Geometry: final body of the model. Coordinates: model frame, mm. Face numbers are marked on the shaded views. A direction names the side the tool comes from. Coordinates: 2 decimals unless noted, no trailing zeros. Write each loop counter-clockwise with the first axis right and the second up, starting at its lowest first coordinate (ties: lowest second). Pieces come first, ordered by that corner, then holes.
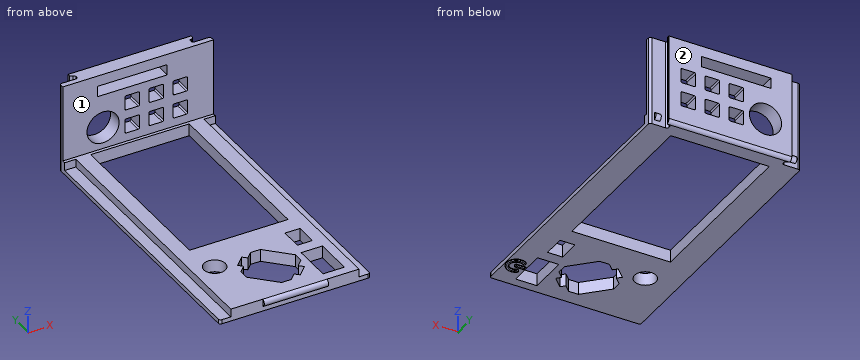
from build123d import *

# Parameters (mm, degrees)
SKETCH_2_W                     = 2.80320188
SKETCH_2_H                     = 4.10319928
SKETCH_2_R                     = 2
SKETCH_2_W_2                   = 3.99999908
SKETCH_2_H_2                   = 7.20319816
EXTRUDE_1_DEPTH                = 2.3
EXTRUDE_2_DEPTH                = 14.4
EXTRUDE_2_DEPTH_BACK           = 2.3
SKETCH_3_W                     = 28.14
SKETCH_3_H                     = 3.4
SKETCH_4_R                     = 3
CUT_EXTRUDE_1_DEPTH            = 3.4
SKETCH_2_3_W                   = 2.1
SKETCH_2_3_H                   = 50.95
CUT_EXTRUDE_2_DEPTH            = 1.5
CUT_EXTRUDE_3_REACH            = 62.506
SKETCH_7_W                     = 28.14
SKETCH_7_H                     = 0.6
SKETCH_8_W                     = 13
SKETCH_8_H                     = 2
CUT_EXTRUDE_4_DEPTH            = 2.8
CUT_EXTRUDE_5_DEPTH            = 16.7
EXTRUDE_3_DEPTH                = 1
EXTRUDE_4_DEPTH                = 6
EXTRUDE_4_DEPTH_BACK           = 6
FILLET_1_R                     = 0.4
FILLET_2_R                     = 0.7
FILLET_3_R                     = 0.4
SKETCH_12_W                    = 2.753
SKETCH_12_H                    = 2.75
CUT_EXTRUDE_6_DEPTH            = 2.8
FILLET_4_R                     = 0.25
PATTERN_LINEAR_1_COUNT         = 3
PATTERN_LINEAR_1_PITCH         = 4.5
PATTERN_LINEAR_1_COUNT_DIR2    = 2
PATTERN_LINEAR_1_PITCH_DIR2    = 4.5
FILLET_4_OF_PATTERN_LINEAR_1_R = 0.25
EXTRUDE_5_DEPTH                = 0.3
FILLET_6_R                     = 0.3
FILLET_5_R                     = 0.15


with BuildPart() as part:
    # 草图2 → 凸台-拉伸1 (new body)
    with BuildSketch(Plane.XY):
        Polygon((-0.1, 0), (-0.1, -50.95), (28.04, -50.95), (28.04, 0), (23.17, 0), (23.17, -32.5), (4.77, -32.5), (4.77, 0), align=None)
        with Locations((22.14500143, -37.80800287)):
            Rectangle(SKETCH_2_W, SKETCH_2_H, mode=Mode.SUBTRACT)
        with Locations((5.9182, -38.735)):
            Circle(SKETCH_2_R, mode=Mode.SUBTRACT)
        Polygon((19.066193866, -43.992617401), (17.88030086, -45.178511502), (18.608616214, -45.906826856), (16.798423264, -47.717019806), (16.070108746, -46.988705288), (14.884217409, -48.174597721), (13.055787589, -48.174595399), (8.873804338, -43.992612148), (8.873804338, -42.164191444), (10.05969962, -40.978296162), (9.331380194, -40.249976736), (11.141573144, -38.439783786), (11.86989257, -39.168103212), (13.055787589, -37.982208193), (14.884217273, -37.982205871), (19.066193866, -42.164182464), align=None, mode=Mode.SUBTRACT)
        with Locations((22.16999884, -45.67000137)):
            Rectangle(SKETCH_2_W_2, SKETCH_2_H_2, mode=Mode.SUBTRACT)
    extrude(amount=-EXTRUDE_1_DEPTH)

    # 草图3 → 凸台-拉伸2 (add, two sides: drawn at the far end of the back side and taken through both)
    with BuildSketch(Plane.XY.offset(-EXTRUDE_2_DEPTH_BACK)):
        with Locations((13.97, 1.7)):
            Rectangle(SKETCH_3_W, SKETCH_3_H)
    extrude(amount=EXTRUDE_2_DEPTH + EXTRUDE_2_DEPTH_BACK)

    # 草图4 → 切除-拉伸1 (cut)
    with BuildSketch(Plane(origin=(0, 3.4, 0), x_dir=(1, 0, 0), z_dir=(0, 1, 0))):
        with Locations(Location((7.41680127, -4.1, 0), (0, 0, 270))):
            Circle(SKETCH_4_R)
    extrude(amount=-CUT_EXTRUDE_1_DEPTH, mode=Mode.SUBTRACT)

    # 草图2<3> → 切除-拉伸2 (cut)
    with BuildSketch(Plane.XY):
        with Locations((0.95, -25.475)):
            Rectangle(SKETCH_2_3_W, SKETCH_2_3_H)
        with Locations((26.99, -25.475)):
            Rectangle(SKETCH_2_3_W, SKETCH_2_3_H)
    extrude(amount=-CUT_EXTRUDE_2_DEPTH, mode=Mode.SUBTRACT)

    # 切除-拉伸3: up to this face of the body (flat: up to its plane)
    cut_extrude_3_end = Plane(part.part.faces().sort_by_distance((13.97, -33.062941036, 0))[0])
    # 草图7 → 切除-拉伸3 (cut, up to the picked face)
    with BuildSketch(Plane.XY.offset(14.4), mode=Mode.PRIVATE) as cut_extrude_3_sk1:
        with Locations((13.97, 0.3)):
            Rectangle(SKETCH_7_W, SKETCH_7_H)
    cut_extrude_3_tool1 = split(extrude(cut_extrude_3_sk1.sketch, amount=-CUT_EXTRUDE_3_REACH, mode=Mode.PRIVATE), bisect_by=cut_extrude_3_end, keep=Keep.BOTH, mode=Mode.PRIVATE)
    add(cut_extrude_3_tool1.solids().sort_by(Axis((13.97, 0.3, 14.4), (0, 0, -1)))[0], mode=Mode.SUBTRACT)

    # 草图8 → 切除-拉伸4 (cut)
    with BuildSketch(Plane.XZ.offset(-0.6)):
        with Locations((12.9, 11.4)):
            Rectangle(SKETCH_8_W, SKETCH_8_H)
    extrude(amount=-CUT_EXTRUDE_4_DEPTH, mode=Mode.SUBTRACT)

    # 草图9 → 切除-拉伸5 (cut)
    with BuildSketch(Plane.XY.offset(14.4)):
        Polygon((2.5, 2.6), (3.3, 2.6), (3.3, 1.6), (-0.1, 1.6), (-0.1, 3.4), (2.5, 3.4), align=None)
        Polygon((28.04, 3.4), (25.44, 3.4), (25.44, 2.6), (24.64, 2.6), (24.64, 1.6), (28.04, 1.6), align=None)
    extrude(amount=-CUT_EXTRUDE_5_DEPTH, mode=Mode.SUBTRACT)

    # 草图10 → 凸台-拉伸3 (add)
    with BuildSketch(Plane.ZY.offset(-0.8)):
        with BuildLine():
            Line((-1.4, 1.6), (0, 1.6))
            ThreePointArc((0, 1.6), (-0.7, 2.1), (-1.4, 1.6))
        make_face()
    extrude_3 = extrude(amount=-EXTRUDE_3_DEPTH)

    # 镜向1: 凸台-拉伸3 across plane
    add(extrude_3.mirror(Plane.ZY.offset(-13.97)))

    # 草图11 → 凸台-拉伸4 (add, two sides: drawn at the far end of the back side and taken through both)
    with BuildSketch(Plane.ZY.offset(-13.97).offset(-EXTRUDE_4_DEPTH_BACK)):
        with BuildLine():
            Line((-1.4, -50.95), (0, -50.95))
            ThreePointArc((0, -50.95), (-0.7, -51.45), (-1.4, -50.95))
        make_face()
    extrude(amount=EXTRUDE_4_DEPTH + EXTRUDE_4_DEPTH_BACK)

    # 圆角1
    fillet_1_edges = [part.edges().sort_by_distance(p)[0] for p in [
        (3.3, 1.6, 6.05),
        (3.3, 2.6, 6.05),
        (2.5, 2.6, 6.05),
        (24.64, 1.6, 6.05),
        (24.64, 2.6, 6.05),
        (25.44, 2.6, 6.05),
    ]]
    fillet(fillet_1_edges, radius=FILLET_1_R - 0.0001)  # a hair under: the kernel refuses the full size

    # 圆角2
    fillet_2_edges = [part.edges().sort_by_distance(p)[0] for p in [
        (13.97, 3.4, -2.3),
    ]]
    fillet(fillet_2_edges, radius=FILLET_2_R)

    # 圆角3
    fillet_3_edges = [part.edges().sort_by_distance(p)[0] for p in [
        (28.04, 1.6, 6.05),
        (-0.1, 1.6, 6.05),
        (-0.1, -50.95, -1.9),
        (28.04, -50.95, -1.9),
    ]]
    fillet(fillet_3_edges, radius=FILLET_3_R)

    # 草图12 → 切除-拉伸6 (cut)
    with BuildSketch(Plane(origin=(0, 3.4, 0), x_dir=(1, 0, 0), z_dir=(0, 1, 0))):
        with Locations((21.8635, -2.975)):
            Rectangle(SKETCH_12_W, SKETCH_12_H)
    cut_extrude_6 = extrude(amount=-CUT_EXTRUDE_6_DEPTH, mode=Mode.SUBTRACT)

    # 圆角4
    fillet_4_edges = [part.edges().sort_by_distance(p)[0] for p in [
        (23.24, 2, 1.6),
        (23.24, 2, 4.35),
        (20.487, 2, 4.35),
        (20.487, 2, 1.6),
    ]]
    fillet(fillet_4_edges, radius=FILLET_4_R)

    # 阵列(线性)1: Cut-Extrude 6 3 × 2
    with Locations(*[(-i * PATTERN_LINEAR_1_PITCH, 0, j * PATTERN_LINEAR_1_PITCH_DIR2) for i in range(PATTERN_LINEAR_1_COUNT) for j in range(PATTERN_LINEAR_1_COUNT_DIR2) if (i, j) != (0, 0)]):
        add(cut_extrude_6, mode=Mode.SUBTRACT)

    # 圆角4 of 阵列(线性)1
    fillet_4_of_pattern_linear_1_edges = [part.edges().sort_by_distance(p)[0] for p in [
        (23.24, 2, 6.1),
        (23.24, 2, 8.85),
        (20.487, 2, 8.85),
        (20.487, 2, 6.1),
        (18.74, 2, 1.6),
        (18.74, 2, 4.35),
        (15.987, 2, 4.35),
        (15.987, 2, 1.6),
        (18.74, 2, 6.1),
        (18.74, 2, 8.85),
        (15.987, 2, 8.85),
        (15.987, 2, 6.1),
        (14.24, 2, 1.6),
        (14.24, 2, 4.35),
        (11.487, 2, 4.35),
        (11.487, 2, 1.6),
        (14.24, 2, 6.1),
        (14.24, 2, 8.85),
        (11.487, 2, 8.85),
        (11.487, 2, 6.1),
    ]]
    fillet(fillet_4_of_pattern_linear_1_edges, radius=FILLET_4_OF_PATTERN_LINEAR_1_R)

    # 草图13 → 凸台-拉伸5 (add)
    with BuildSketch(Plane(origin=(0, 0, -2.3), x_dir=(-1, 0, 0), z_dir=(0, 0, -1))):
        with BuildLine():
            Line((-25.256471053, -44.821473233), (-24.832206984, -44.397209164))
            ThreePointArc((-24.832206984, -44.397209164), (-27.90499919, -45.67000137), (-24.832206984, -46.942793576))
            Line((-24.832206984, -46.942793576), (-25.256471053, -46.518529507))
            ThreePointArc((-25.256471053, -46.518529507), (-27.30499919, -45.67000137), (-25.256471053, -44.821473233))
        make_face()
        with BuildLine():
            Line((-26.10499919, -45.37000137), (-24.60499919, -45.37000137))
            ThreePointArc((-24.60499919, -45.37000137), (-24.30499919, -45.67000137), (-24.60499919, -45.97000137))
            Line((-24.60499919, -45.97000137), (-26.10499919, -45.97000137))
            ThreePointArc((-26.10499919, -45.97000137), (-26.40499919, -45.67000137), (-26.10499919, -45.37000137))
        make_face()
    extrude(amount=EXTRUDE_5_DEPTH)

    # 圆角6
    fillet_6_edges = [part.edges().sort_by_distance(p)[0] for p in [
        (24.832206984, -46.942793576, -2.45),
        (25.256471053, -46.518529507, -2.45),
        (25.256471053, -44.821473233, -2.45),
        (24.832206984, -44.397209164, -2.45),
    ]]
    fillet(fillet_6_edges, radius=FILLET_6_R - 0.0001)  # a hair under: the kernel refuses the full size

    # 圆角5
    fillet_5_edges = [part.edges().sort_by_distance(p)[0] for p in [
        (26.40499919, -45.67000137, -2.6),
        (25.35499919, -45.97000137, -2.6),
        (24.30499919, -45.67000137, -2.6),
        (25.35499919, -45.37000137, -2.6),
        (27.90499919, -45.67000137, -2.6),
        (27.30499919, -45.67000137, -2.6),
        (24.979360848, -44.388492506, -2.6),
        (25.247753249, -44.717149471, -2.6),
        (25.247753249, -46.622853269, -2.6),
        (24.979360848, -46.951510234, -2.6),
    ]]
    fillet(fillet_5_edges, radius=FILLET_5_R)


solid = part.part
Item 1: Section B-B, the plane y = -3. Output: boundary loops of the cut face in (x, z).
Derived:
outline: (-0.1, -2.3) - (4.77, -2.3) - (4.77, 0) - (2, 0) - (2, -1.5) - (-0.1, -1.5) - close; (23.17, -2.3) - (28.04, -2.3) - (28.04, -1.5) - (25.94, -1.5) - (25.94, 0) - (23.17, 0) - close
Item 2: Pin query (flat end, axial travel): pin 1 (5 mm diameter, centred on y = -2, z = 12.5, fed in from +X); pin 2 (5 mm diameter, centred on x = 21, y = -29.5, fed in from +Z); pin 3 (6 mm diameter, centred on x = 14, z = 7.5, fed in from -Y); pin 4 (6.5 mm diameter, centred on x = 5.92, y = -38.74, fed in from -Z). Return the tip coordinate at first contact, or that it passes through.
Derived:
pin 1: passes through
pin 2: stops at z = 0
pin 3: stops at y = 0.6
pin 4: stops at z = -2.3
Item 3: Section A-A, the plane x = 22. Output: boundary loops of the cut face in (y, z).
Derived:
outline: (-50.95, -2.3) - (-49.27, -2.3) - (-49.27, 0) - (-50.95, 0) - close; (-42.07, -2.3) - (-39.86, -2.3) - (-39.86, 0) - (-42.07, 0) - close; (-35.76, -2.3) - (-32.5, -2.3) - (-32.5, 0) - (-35.76, 0) - close; (0, -2.3) - (2.7, -2.3) arc R0.7 ccw to (3.4, -1.6) - (3.4, 1.6) - (0.6, 1.6) - (0.6, 0) - (0, 0) - close; (0.6, 4.35) - (3.4, 4.35) - (3.4, 6.1) - (0.6, 6.1) - close; (0.6, 8.85) - (3.4, 8.85) - (3.4, 14.4) - (0.6, 14.4) - close
Item 4: Section C-C, the plane y = -33.5. Output: boundary loops of the cut face in (x, z), plus the area to 3 significant figures.
Derived:
outline: (-0.1, -2.3) - (28.04, -2.3) - (28.04, -1.5) - (25.94, -1.5) - (25.94, 0) - (2, 0) - (2, -1.5) - (-0.1, -1.5) - close
area: 58.4 mm2
Item 5: Material intervals for probe 1 along X at (y, z) = (1.9, 4.1); probe 2 along Z at (x, y) = (22.5, 1.5); probe 3 along X at (y, z) = (1.8, 4.1), sorted ascending.
Derived:
probe 1: x = 3.29 to 4.42, 10.42 to 11.49, 14.24 to 15.99, 18.74 to 20.49, 23.24 to 24.65
probe 2: z = -2.3 to 1.6, 4.35 to 6.1, 8.85 to 14.4
probe 3: x = 3.25 to 4.42, 10.42 to 11.49, 14.24 to 15.99, 18.74 to 20.49, 23.24 to 24.69
Item 6: Section D-D, the plane z = 2.75. State how many separate pieces and enclosed holes the cut face has, plus the area to 3 significant figures.
Derived:
separate pieces: 5
enclosed holes: 0
area: 29.7 mm2
Item 7: Set-up query: the marked faces 1 and 2. Return all of +Z, -Z, +X, -X, +Y, -Y with unobstructed straight access to the full face (end or side cutting, diameter ignored); none if empty.
Derived:
face 1: +Z, +X, -X, -Y
face 2: +Z, -Z, +X, -X, +Y
